Read the model definition and answer for the solid it produces. Units are mm, in the model's axes. Face numbers are marked on the shaded views. Give positions to 0.01 mm unless a question says otherwise; leave off trailing zeros. Order: outer loops, then holes, each group sorted by start corner. A loop starts at its lowest first (then second) coordinate and runs counter-clockwise, first axis right, second up. Notation, with made-up numbers: (-32, 37.25) - (-3, 37.25) arc R22 cw to (-3, 45.25) - close; hole circle Ø8 at (71, 55). An arc over 180 degrees is marked (long way). Answer as CSV lines item,"result". Start each with the question number.
from build123d import *

# Parameters (mm, degrees)
F1_DEPTH = 35
F2_R     = 5
F3_DEPTH = 52.2


with BuildPart() as f1:
    # F0 (on Front) → F1 (new body)
    with BuildSketch(Plane.XZ):
        Polygon((3.207181, 5.555), (-3.207181, 5.555), (-6.414361, 0), (-3.207181, -5.555), (3.207181, -5.555), (6.414361, 0), align=None)
    extrude(amount=F1_DEPTH)

    # F2 (on Front) → F3 (cut)
    with BuildSketch(Plane.XZ):
        Circle(F2_R)
    extrude(amount=F3_DEPTH, mode=Mode.SUBTRACT)


solid = f1.part
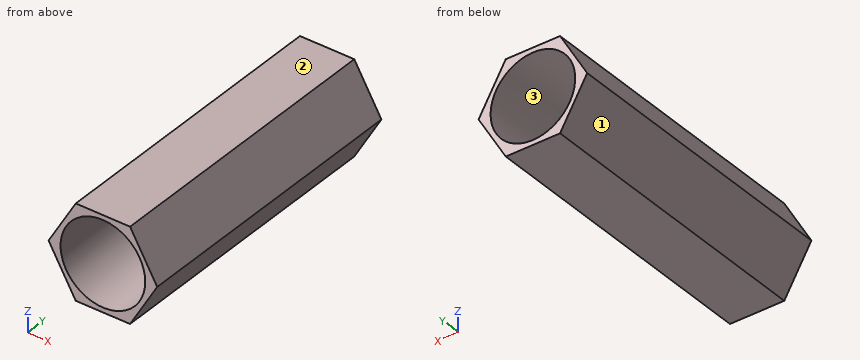
(1) Section A-A, the plane x = 0 is taken. Write down the section's boundary in (y, z) (3 decimals).
(2) Determine the mould class of the marked faces 1, 2 and 3 for opening direction X: released by +X, released by -X, zero draft, split by the parting line, or undercut.
(3) Section B-B, the plane z = -2.25 is taken. Write down the section's boundary in (x, y).
(4) Flat-ended cylindrical pins translate along their axes: pin 1 Ø1.5 at (y, z) = (-16, -1.5) entering from +X; pin 2 Ø4 at (x, z) = (-2.5, -1) entering from +Y. Find the tip coordinate at first contact, or state that the pin passes through.
(5) Straight lines are drawn through the part: line 1 (Z direction, x = 0, y = -24) (3 decimals); line 2 (Z direction, x = -4, y = -23.5); line 3 (X direction, y = -18, z = 3). For each, find the intervals that lie inside material, in ascending order. Write a range as [from, to].
(6) Section C-C, the plane y = -26.5 is taken. Write down the section's boundary in (x, z) (3 decimals), and give its area (3 significant figures).
Checks:
1,outline,"(-35, -5.555) - (0, -5.555) - (0, -5) - (-35, -5) - close; (-35, 5) - (0, 5) - (0, 5.555) - (-35, 5.555) - close"
2,face 1,"released by -X"
2,face 2,"zero draft"
2,face 3,"undercut"
3,outline,"(-5.12, -35) - (-4.47, -35) - (-4.47, 0) - (-5.12, 0) - close; (4.47, -35) - (5.12, -35) - (5.12, 0) - (4.47, 0) - close"
4,pin 1,"stops at x = 5.98"
4,pin 2,"passes through"
5,line 1,"z = [-5.555, -5], [5, 5.555]"
5,line 2,"z = [-4.18, -3], [3, 4.18]"
5,line 3,"x = [-4.68, -4], [4, 4.68]"
6,outline,"(-6.414, 0) - (-3.207, -5.555) - (3.207, -5.555) - (6.414, 0) - (3.207, 5.555) - (-3.207, 5.555) - close; hole circle Ø10 at (0, 0)"
6,area,"28.4 mm²"
